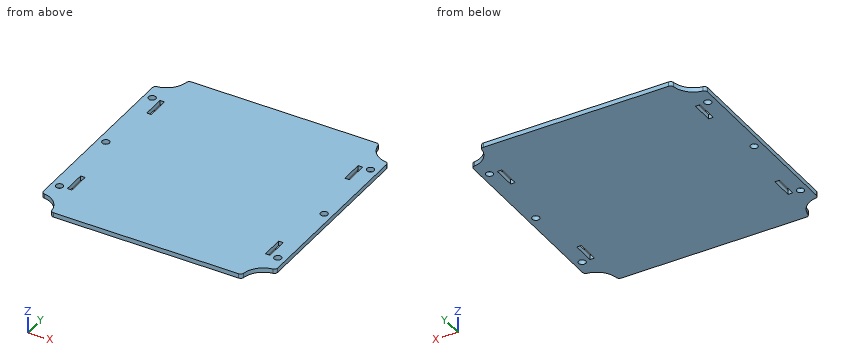
```python
from build123d import *

# Parameters (mm, degrees)
CROQUIS1_R              = 1.6
CROQUIS1_W              = 2
CROQUIS1_H              = 10
SALIENTE_EXTRUIR1_DEPTH = 2


with BuildPart() as part:
    # Croquis1 → Saliente-Extruir1 (new body)
    with BuildSketch(Plane.XY):
        with BuildLine():
            Line((10.897247359, 0), (93.102752641, 0))
            ThreePointArc((93.102752641, 0), (94.088445752, 0.369332458), (94.588740917, 1.295454545))
            ThreePointArc((94.588740917, 1.295454545), (97.282485579, 6.717514421), (102.704545455, 9.411259083))
            ThreePointArc((102.704545455, 9.411259083), (103.630667542, 9.911554248), (104, 10.897247359))
            Line((104, 10.897247359), (104, 93.102752641))
            ThreePointArc((104, 93.102752641), (103.630667542, 94.088445752), (102.704545455, 94.588740917))
            ThreePointArc((102.704545455, 94.588740917), (97.282485579, 97.282485579), (94.588740917, 102.704545455))
            ThreePointArc((94.588740917, 102.704545455), (94.088445752, 103.630667542), (93.102752641, 104))
            Line((93.102752641, 104), (10.897247359, 104))
            ThreePointArc((10.897247359, 104), (9.911554248, 103.630667542), (9.411259083, 102.704545455))
            ThreePointArc((9.411259083, 102.704545455), (6.717514421, 97.282485579), (1.295454545, 94.588740917))
            ThreePointArc((1.295454545, 94.588740917), (0.369332458, 94.088445752), (0, 93.102752641))
            Line((0, 93.102752641), (0, 10.897247359))
            ThreePointArc((0, 10.897247359), (0.369332458, 9.911554248), (1.295454545, 9.411259083))
            ThreePointArc((1.295454545, 9.411259083), (6.717514421, 6.717514421), (9.411259083, 1.295454545))
            ThreePointArc((9.411259083, 1.295454545), (9.911554248, 0.369332458), (10.897247359, 0))
        make_face()
        with Locations((3.5, 52)):
            Circle(CROQUIS1_R, mode=Mode.SUBTRACT)
        with Locations((3.5, 87)):
            Circle(CROQUIS1_R, mode=Mode.SUBTRACT)
        with Locations(Location((3.5, 17, 0), (0, 0, 180))):
            Circle(CROQUIS1_R, mode=Mode.SUBTRACT)
        with Locations((100.5, 17)):
            Circle(CROQUIS1_R, mode=Mode.SUBTRACT)
        with Locations(Location((100.5, 52, 0), (0, 0, 180))):
            Circle(CROQUIS1_R, mode=Mode.SUBTRACT)
        with Locations(Location((100.5, 87, 0), (0, 0, 180))):
            Circle(CROQUIS1_R, mode=Mode.SUBTRACT)
        with Locations((8, 82)):
            Rectangle(CROQUIS1_W, CROQUIS1_H, mode=Mode.SUBTRACT)
        with Locations((96, 82)):
            Rectangle(CROQUIS1_W, CROQUIS1_H, mode=Mode.SUBTRACT)
        with Locations((96, 22)):
            Rectangle(CROQUIS1_W, CROQUIS1_H, mode=Mode.SUBTRACT)
        with Locations((8, 22)):
            Rectangle(CROQUIS1_W, CROQUIS1_H, mode=Mode.SUBTRACT)
    extrude(amount=-SALIENTE_EXTRUIR1_DEPTH)


solid = part.part
```
For this review, take the finished solid that the model builds, in its own axes (mm). Round coordinates to 2 decimals unless told otherwise and drop trailing zeros. Write each loop counter-clockwise with the first axis right and the second up, starting at its lowest first coordinate (ties: lowest second). Pieces come first, ordered by that corner, then holes. Notation, with made-up numbers: M 78.25,56 L 137.25,56 A19 cw 137.25,88 Z; hole C 76,47 d6. An arc over 180 degrees is marked long. One line per item, written item: value. Start each with the question number.
(1) Wall thickness on line 1 (X direction, y = 78.5, z = -0.1); line 2 (X direction, y = 86, z = -0.35); line 3 (Y direction, x = 3.5, z = -0.45): over which ranges is each line inside the solid? List them lowest first.
(2) We need section A-A (y = 52). Give the boundary of the cut face in (x, z).
(3) Insertion check: pin 1 (0.6 mm diameter, centred on x = 8, z = -1.5, fed in from -Y); pin 2 (5 mm diameter, centred on x = 100.5, y = 52, fed in from +Z); pin 3 (3 mm diameter, centred on x = 100.5, y = 17, fed in from -Z). Each pin has a flat end and moves straight along its axis. Give the tip position at first contact, or say it passes through.
(4) We need section C-C (z = -1.3). Count the separate pieces of the cut face and the enclosed holes in it, and give its area (3 significant figures).
(5) We need section B-B (x = 3.5). Give the boundary of the cut face in (y, z), and give its area (3 significant figures).
Result:
1. line 1: 0 to 7, 9 to 95, 97 to 104
1. line 2: 0 to 2.25, 4.75 to 7, 9 to 95, 97 to 99.25, 101.75 to 104
1. line 3: 8.83 to 15.4, 18.6 to 50.4, 53.6 to 85.4, 88.6 to 95.17
2. outline: M 0,-2 L 1.9,-2 L 1.9,0 L 0,0 Z; M 5.1,-2 L 98.9,-2 L 98.9,0 L 5.1,0 Z; M 102.1,-2 L 104,-2 L 104,0 L 102.1,0 Z
3. pin 1: y = 4.62
3. pin 2: z = 0
3. pin 3: through
4. separate pieces: 1
4. enclosed holes: 10
4. area: 10,400 mm²
5. outline: M 8.83,-2 L 15.4,-2 L 15.4,0 L 8.83,0 Z; M 18.6,-2 L 50.4,-2 L 50.4,0 L 18.6,0 Z; M 53.6,-2 L 85.4,-2 L 85.4,0 L 53.6,0 Z; M 88.6,-2 L 95.17,-2 L 95.17,0 L 88.6,0 Z
5. area: 153 mm²
